Source: CAD feature listing. Evaluate the final solid. Frame: model axes, mm. A direction names the side the tool comes from. Round coordinates to 2 decimals unless told otherwise and drop trailing zeros. Loops run counter-clockwise (first coordinate to the right, second up) from the corner with the lowest first, then second, coordinate; pieces in that order, holes last. Notation, with made-up numbers: (-2.5, 45.25) - (45.5, 45.25) arc R20 cw to (45.5, 79.25) - close; hole circle Ø7 at (-19, 80). An arc over 180 degrees is marked (long way). Write item = value, one per line. Start each with the question number.
from build123d import *

# Parameters (mm, degrees)
SKETCH_1_R               = 10
EXTRUDE_1_DEPTH          = 20
SKETCH_2_R               = 9
EXTRUDE_2_DEPTH          = 8
SKETCH_3_R               = 3
CUT_EXTRUDE_1_DEPTH      = 11
CUT_EXTRUDE_1_DEPTH_BACK = 11
FILLET_1_R               = 0.5
CHAMFER_1_SIZE           = 0.5


with BuildPart() as part:
    # 草图1 → 凸台-拉伸1 (new body)
    with BuildSketch(Plane(origin=(0, 0, 0), x_dir=(1, 0, 0), z_dir=(0, 1, 0))):
        Circle(SKETCH_1_R)
    extrude(amount=EXTRUDE_1_DEPTH)

    # 草图2 → 凸台-拉伸2 (add)
    with BuildSketch(Plane.XZ):
        Circle(SKETCH_2_R)
    extrude(amount=EXTRUDE_2_DEPTH)

    # 草图3 → 切除-拉伸1 (cut, two sides)
    with BuildSketch(Plane.XY) as cut_extrude_1_sk:
        with Locations((0, 13)):
            Circle(SKETCH_3_R)
    extrude(amount=CUT_EXTRUDE_1_DEPTH, mode=Mode.SUBTRACT)
    extrude(cut_extrude_1_sk.sketch, amount=-CUT_EXTRUDE_1_DEPTH_BACK, mode=Mode.SUBTRACT)

    # 圆角1
    fillet_1_edges = [part.edges().sort_by_distance(p)[0] for p in [
        (-10, 0, 0),
    ]]
    fillet(fillet_1_edges, radius=FILLET_1_R)

    # 倒角1
    chamfer_1_edges = [part.edges().sort_by_distance(p)[0] for p in [
        (-9, -8, 0),
    ]]
    chamfer(chamfer_1_edges, length=CHAMFER_1_SIZE)


solid = part.part
(1) Cut plane A-A (x = 0). Output: boundary loops of the cut face in (y, z).
(2) Cut plane B-B (y = 6). Output: boundary loops of the cut face in (x, z), and give its area (3 significant figures).
(3) Access query for faces 1 (the face through (0, 20, 0)), 2 (the face through (-6, 0, 7)). Directions: +Z, -Z, +X, -X, +Y, -Y. A direction counts if a zero-diameter tool reaches every point of the face in a straight line with its end or side. Return the directions, or none.
(4) Pin query (flat end, axial travel): P1, Ø6, axis at x = 7, y = -3.5, coming from the +Z side; P2, Ø3, axis at x = -5, y = 7, coming from the -Z side; P3, Ø1, axis at x = 3.5, y = 14.5, coming from the +Z side; P4, Ø9.5, axis at x = 0, y = 13, coming from the +Z side. Return the tip coordinate at first contact, or that it passes through.
(5) Material intervals for line 1 along Y through (x, z) = (0, -1.75); line 2 along Y through (x, z) = (1.25, -2); line 3 along X through (y, z) = (12.75, -8.75), sorted ascending. Write a range as from..to.
(6) Cut plane D-D (y = -4). Output: boundary loops of the cut face in (x, z).
(7) Cut plane C-C (y = 13). Output: boundary loops of the cut face in (x, z), and give its area (3 significant figures).
Solution:
q1.outline = (-8, -8.5) - (-7.5, -9) - (0, -9) - (0, -9.5) arc R0.5 ccw to (0.5, -10) - (10, -10) - (10, 10) - (0.5, 10) arc R0.5 ccw to (0, 9.5) - (0, 9) - (-7.5, 9) - (-8, 8.5) - close; (16, -10) - (20, -10) - (20, 10) - (16, 10) - close
q2.outline = circle Ø20 at (0, 0)
q2.area = 314 mm^2
q3.face_1 = +Z, -Z, +X, -X, +Y
q3.face_2 = -Y
q4.P1 = 8.06
q4.P2 = -9.37
q4.P3 = 9.54
q4.P4 = 10
q5.line_1 = -8..10, 16..20
q5.line_2 = -8..10.27, 15.73..20
q5.line_3 = -4.84..-2.99, 2.99..4.84
q6.outline = circle Ø18 at (0, 0)
q7.outline = (-3, -9.54) - (-3, 9.54) arc R10 ccw to start; (3, -9.54) arc R10 ccw to (3, 9.54) - close
q7.area = 196 mm^2
